The model under review builds one solid part; all positions refer to its coordinate system, in mm. A direction names the side the tool comes from. Give positions to 0.01 mm unless a question says otherwise; leave off trailing zeros. Loops run counter-clockwise (first coordinate to the right, second up) from the corner with the lowest first, then second, coordinate; pieces in that order, holes last. Notation, with made-up numbers: M 84.25,-6.75 L 113.25,-6.75 A33 ccw 113.25,25.25 Z; hole C -8.5,78 d9. An arc over 180 degrees is marked long. Return JSON: item names as keys, results as strings.
```python
from build123d import *

# Parameters (mm, degrees)
F0_W     = 50.8
F0_H     = 304.8
F1_DEPTH = 101.6


# Not quite as in the source:
# - a feature names something its author has since deleted; it is built from what else it names


with BuildPart() as f1:
    # F0 (on Top) → F1 (new body)
    with BuildSketch(Plane.XY):
        Polygon((422.6718741447, 202.9749498913), (371.8718741447, 202.9749498913), (371.8718741447, 152.1749498913), (371.8718741447, -152.6250501087), (371.8718741447, -204.3104916811), (422.6718741447, -204.3104916811), align=None)
        Polygon((-110.7281258553, -152.6250501087), (-110.7281258553, 152.1749498913), (-110.7281258553, 202.9749498913), (-161.5281258553, 202.9749498913), (-161.5281258553, -152.6250501087), (-161.5281258553, -203.4250501087), (-110.7281258553, -203.4250501087), align=None)
        Polygon((-110.7281258553, 202.9749498913), (-110.7281258553, 152.1749498913), (16.2718741447, 152.1749498913), (67.0718741447, 152.1749498913), (194.0718741447, 152.1749498913), (244.8718741447, 152.1749498913), (371.8718741447, 152.1749498913), (371.8718741447, 202.9749498913), align=None)
        with Locations((41.6718741447, -0.2250501087)):
            Rectangle(F0_W, F0_H)
        with Locations((219.4718741447, -0.2250501087)):
            Rectangle(F0_W, F0_H)
        Polygon((16.2718741447, -152.6250501087), (-110.7281258553, -152.6250501087), (-110.7281258553, -203.4250501087), (371.8718741447, -204.3104916811), (371.8718741447, -152.6250501087), (244.8718741447, -152.6250501087), (194.0718741447, -152.6250501087), (67.0718741447, -152.6250501087), align=None)
    extrude(amount=F1_DEPTH)


solid = f1.part
```
1) Consider section B-B on y = 43. Write out the cut boundary in (x, z), then the cut area to 3 significant figures.
From the geometry:
{"outline": "M -161.53,0 L -110.73,0 L -110.73,101.6 L -161.53,101.6 Z; M 16.27,0 L 67.07,0 L 67.07,101.6 L 16.27,101.6 Z; M 194.07,0 L 244.87,0 L 244.87,101.6 L 194.07,101.6 Z; M 371.87,0 L 422.67,0 L 422.67,101.6 L 371.87,101.6 Z", "area": "20,600 mm²"}
2) Consider section C-C on x = 325.5. Write out the cut boundary in (y, z), then the cut area to 3 significant figures.
From the geometry:
{"outline": "M -204.23,0 L -152.63,0 L -152.63,101.6 L -204.23,101.6 Z; M 152.17,0 L 202.97,0 L 202.97,101.6 L 152.17,101.6 Z", "area": "10,400 mm²"}
3) Consider section A-A on z = 49.5. Write out the cut boundary in (x, y).
From the geometry:
{"outline": "M -161.53,-203.43 L -110.73,-203.43 L 371.87,-204.31 L 422.67,-204.31 L 422.67,202.97 L -161.53,202.97 Z; hole M -110.73,-152.63 L 16.27,-152.63 L 16.27,152.17 L -110.73,152.17 Z; hole M 67.07,-152.63 L 194.07,-152.63 L 194.07,152.17 L 67.07,152.17 Z; hole M 244.87,-152.63 L 371.87,-152.63 L 371.87,152.17 L 244.87,152.17 Z"}
4) The part is to be moulded in two halves that separate along X. For faces 4 (the face through (422.672, -4, 50)), 5 (the face through (-161.528, 3, 50)), 6 (the face through (67.072, -2, 50)), 7 (the face through (397, -204.31, 50)), say which applies: released by +X, released by -X, zero draft, split by the parting line, or undercut.
From the geometry:
{"face 4": "released by +X", "face 5": "released by -X", "face 6": "undercut", "face 7": "zero draft"}
5) Consider section D-D on x = 183. Write out the cut boundary in (y, z), then the cut area to 3 significant figures.
From the geometry:
{"outline": "M -203.96,0 L -152.63,0 L -152.63,101.6 L -203.96,101.6 Z; M 152.17,0 L 202.97,0 L 202.97,101.6 L 152.17,101.6 Z", "area": "10,400 mm²"}
6) Tool access review of faces 1 (the face through (244.872, -2, 50)), 2 (the face through (-136, -203.425, 50)), 3 (the face through (62, 2, 101.6)): name each direction out of +Z, -Z, +X, -X, +Y, -Y from which nothing blocks a thin tool from reaching the whole face with its end or side.
From the geometry:
{"face 1": "+Z, -Z", "face 2": "+Z, -Z, -X, -Y", "face 3": "+Z, +X, -X, +Y, -Y"}
7) Wall thickness on L1, parallel to X at y = 79, z = 12.5; L2, parallel to Y at x = 300, z = 28; L3, parallel to Y at x = -47.5, z = 26: over which ranges is each line inside the solid? List them lowest first. Write a range as from..to.
From the geometry:
{"L1": "-161.53..-110.73, 16.27..67.07, 194.07..244.87, 371.87..422.67", "L2": "-204.18..-152.63, 152.17..202.97", "L3": "-203.54..-152.63, 152.17..202.97"}
8) Insertion check: pin 1 (1 mm diameter, centred on x = 343.5, z = 26, fed in from -Y). The pin has a flat end and moves straight along its axis. Give the tip position at first contact, or say it passes through.
From the geometry:
{"pin 1": "y = -204.26"}
